```python
from build123d import *

# Parameters (mm, degrees)
BOSS_EXTRUDE1_DEPTH = 3.175
SKETCH4_R           = 3
SKETCH4_R_2         = 1.5
CUT_EXTRUDE1_DEPTH  = 181.721002169
SKETCH5_R           = 4.25
CUT_EXTRUDE2_DEPTH  = 181.721002169
SKETCH10_R          = 1.5
CUT_EXTRUDE4_DEPTH  = 181.721002169
FILLET1_R           = 10
FILLET2_R           = 10
SKETCH11_R          = 7.75
CUT_EXTRUDE5_DEPTH  = 181.721002169
SKETCH13_R          = 1.75
CUT_EXTRUDE6_DEPTH  = 181.721002169


with BuildPart() as part:
    # Sketch1 → Boss-Extrude1 (new body)
    with BuildSketch(Plane(origin=(0, 0, 0), x_dir=(1, 0, 0), z_dir=(0, 1, 0))):
        Polygon((45, -45), (93.251405711, -22.5), (175, -22.5), (175, 22.5), (93.251405711, 22.5), (45, 45), (-45, 45), (-45, -45), align=None)
    extrude(amount=BOSS_EXTRUDE1_DEPTH)

    # Sketch4 → Cut-Extrude1 (cut, through all)
    with BuildSketch(Plane(origin=(0, 3.175, 0), x_dir=(1, 0, 0), z_dir=(0, 1, 0))):
        with Locations(Location((150, 0, 0), (0, 0, 270))):
            Circle(SKETCH4_R)
        with Locations(Location((136, 9, 0), (0, 0, 270))):
            Circle(SKETCH4_R_2)
        with Locations(Location((164, 9, 0), (0, 0, 90))):
            Circle(SKETCH4_R_2)
        with Locations(Location((164, -9, 0), (0, 0, 270))):
            Circle(SKETCH4_R_2)
        with Locations(Location((136, -9, 0), (0, 0, 90))):
            Circle(SKETCH4_R_2)
    extrude(amount=-CUT_EXTRUDE1_DEPTH, mode=Mode.SUBTRACT)

    # Sketch5 → Cut-Extrude2 (cut, through all)
    with BuildSketch(Plane(origin=(0, 3.175, 0), x_dir=(1, 0, 0), z_dir=(0, 1, 0))):
        with Locations(Location((0, 0, 0), (0, 0, 270))):
            Circle(SKETCH5_R)
    extrude(amount=-CUT_EXTRUDE2_DEPTH, mode=Mode.SUBTRACT)

    # Sketch10 → Cut-Extrude4 (cut, through all)
    with BuildSketch(Plane(origin=(0, 3.175, 0), x_dir=(1, 0, 0), z_dir=(0, 1, 0))):
        with Locations(Location((80.5, -17.5, 0), (0, 0, 270))):
            Circle(SKETCH10_R)
        with Locations(Location((116, -17.5, 0), (0, 0, 270))):
            Circle(SKETCH10_R)
        with Locations(Location((116, 17.5, 0), (0, 0, 90))):
            Circle(SKETCH10_R)
        with Locations(Location((80.5, 17.5, 0), (0, 0, 90))):
            Circle(SKETCH10_R)
    extrude(amount=-CUT_EXTRUDE4_DEPTH, mode=Mode.SUBTRACT)

    # Fillet1
    fillet1_edges = [part.edges().sort_by_distance(p)[0] for p in [
        (-45, 1.5875, 45),
        (-45, 1.5875, -45),
        (175, 1.5875, -22.5),
        (175, 1.5875, 22.5),
    ]]
    fillet(fillet1_edges, radius=FILLET1_R)

    # Fillet2
    fillet2_edges = [part.edges().sort_by_distance(p)[0] for p in [
        (93.251405711, 1.5875, 22.5),
        (45, 1.5875, 45),
        (45, 1.5875, -45),
        (93.251405711, 1.5875, -22.5),
    ]]
    fillet(fillet2_edges, radius=FILLET2_R)

    # Sketch11 → Cut-Extrude5 (cut, through all)
    with BuildSketch(Plane(origin=(0, 3.175, 0), x_dir=(1, 0, 0), z_dir=(0, 1, 0))):
        with Locations(Location((-31.819805153, 31.819805153, 0), (0, 0, 270))):
            Circle(SKETCH11_R)
        with Locations(Location((31.819805153, 31.819805153, 0), (0, 0, 270))):
            Circle(SKETCH11_R)
        with Locations(Location((31.819805153, -31.819805153, 0), (0, 0, 270))):
            Circle(SKETCH11_R)
        with Locations(Location((-31.819805153, -31.819805153, 0), (0, 0, 270))):
            Circle(SKETCH11_R)
    extrude(amount=-CUT_EXTRUDE5_DEPTH, mode=Mode.SUBTRACT)

    # Sketch13 → Cut-Extrude6 (cut, through all)
    with BuildSketch(Plane(origin=(0, 3.175, 0), x_dir=(1, 0, 0), z_dir=(0, 1, 0))):
        with Locations(Location((8, 0, 0), (0, 0, 270))):
            Circle(SKETCH13_R)
        with Locations(Location((0, -8, 0), (0, 0, 270))):
            Circle(SKETCH13_R)
        with Locations(Location((-8, 0, 0), (0, 0, 270))):
            Circle(SKETCH13_R)
        with Locations(Location((0, 8, 0), (0, 0, 270))):
            Circle(SKETCH13_R)
    extrude(amount=-CUT_EXTRUDE6_DEPTH, mode=Mode.SUBTRACT)


solid = part.part
```
CAD build for the part. Positions are in the model's coordinates, mm. Round coordinates to 2 decimals unless told otherwise and drop trailing zeros. Loops run counter-clockwise (first coordinate to the right, second up) from the corner with the lowest first, then second, coordinate; pieces in that order, holes last. Notation, with made-up numbers: M 48.25,38 L 107.25,38 A23 ccw 107.25,47 Z; hole C 52.5,-18.75 d1. An arc over 180 degrees is marked long. Use a Markdown table: item, result. Add a question column.
(1) Pull direction X, two halves, no side cores. Call faces 1 (the face through (39, 0, -1)), 2 (the face through (172.15, 1.61, -19.49)), 3 (the face through (-34.79, 1.61, 38.98)): +X half, -X half, draft (parallel to the pull), parting line (faces both ways), or undercut.
(2) Flat gauge pins, fed straight in: pin 1 (25 mm diameter, centred on x = -31.82, z = -31.82, fed in from -Y); pin 2 (2.5 mm diameter, centred on x = 116, z = 17.5, fed in from +Y); pin 3 (1.5 mm diameter, centred on y = 2, z = -33.5, fed in from +X); pin 4 (1 mm diameter, centred on x = 143.5, y = 1, fed in from -Z). Where does each tip first touch, or does it go through?
(3) Drill centre lines: line 1 (X direction, y = 1.95, z = 0); line 2 (Z direction, x = 136, y = 0.7); line 3 (X direction, y = 0.35, z = 18.5). Where is each one in solid material? Low to high.
(4) Cut at B-B (z = -28). Give the cut face in (x, y) (3 decimals), and give its area (3 significant figures).
(5) Cut at C-C (y = 2.45). State how many separate pieces and enclosed holes the cut face has, and give its area (3 significant figures).
(6) Cut at A-A (x = 150). Give the cut face in (y, z) (3 decimals).
Geometry says:
| question | item | result |
|---|---|---|
| 1 | face 1 | draft |
| 1 | face 2 | +X half |
| 1 | face 3 | undercut |
| 2 | pin 1 | stops at y = 0 |
| 2 | pin 2 | passes through |
| 2 | pin 3 | stops at x = 71.27 |
| 2 | pin 4 | stops at z = -22.5 |
| 3 | line 1 | x = -45 to -9.75, -6.25 to -4.25, 4.25 to 6.25, 9.75 to 147, 153 to 175 |
| 3 | line 2 | z = -22.5 to -10.5, -7.5 to 7.5, 10.5 to 22.5 |
| 3 | line 3 | x = -45 to 79.38, 81.62 to 114.88, 117.12 to 173 |
| 4 | outline | M -45,0 L -38.563,0 L -38.563,3.175 L -45,3.175 Z; M -25.077,0 L 25.077,0 L 25.077,3.175 L -25.077,3.175 Z; M 38.563,0 L 81.457,0 L 81.457,3.175 L 38.563,3.175 Z |
| 4 | area | 316 mm² |
| 5 | separate pieces | 1 |
| 5 | enclosed holes | 18 |
| 5 | area | 14,000 mm² |
| 6 | outline | M 0,-22.5 L 3.175,-22.5 L 3.175,-3 L 0,-3 Z; M 0,3 L 3.175,3 L 3.175,22.5 L 0,22.5 Z |
